Autodesk Inventor part; units mm, degrees
ref_plane "Start plane" through (0, 0, -25) normal (0, 0, 1) x (1, 0, 0)
ref_plane "End plane" through (0, 0, 2335) normal (0, 0, 1) x (1, 0, 0)
ref_plane "Work Plane4" through (0, 21, -25) normal (0, 0, -1) x (-1, 0, 0)
ref_plane "Start plane" through (0, 0, -25) normal (0, 0, 1) x (1, 0, 0)
ref_plane "End plane" through (0, 0, 2335) normal (0, 0, 1) x (1, 0, 0)
sketch "Sketch" plane through (0, 0, 0) normal (0, 0, 1) x (1, 0, 0)
  line L0 (-25, -21) -> (-25, 21)
  line L1 (-21, 25) -> (21, 25)
  line L2 (25, 21) -> (25, -21)
  line L3 (21, -25) -> (-21, -25)
  arc A0 (-25, -21) -> (-21, -25) centre (-21, -21) ccw
  arc A1 (25, 21) -> (21, 25) centre (21, 21) ccw
  arc A2 (-21, 25) -> (-25, 21) centre (-21, 21) ccw
  arc A3 (21, -25) -> (25, -21) centre (21, -21) ccw
  arc A4 (-21, 23) -> (-23, 21) centre (-21, 21) ccw
  line L4 (-21, 23) -> (21, 23)
  arc A5 (23, 21) -> (21, 23) centre (21, 21) ccw
  line L5 (23, 21) -> (23, -21)
  arc A6 (21, -23) -> (23, -21) centre (21, -21) ccw
  line L6 (21, -23) -> (-21, -23)
  arc A7 (-23, -21) -> (-21, -23) centre (-21, -21) ccw
  line L7 (-23, -21) -> (-23, 21)
  line L8 (0, 36.4497) -> (0, -36.4497) construction
  line L9 (-36.4497, 0) -> (36.4497, 0) construction
  dimension "d7" = 4
  dimension "d9" = 50
  dimension "d11" = 50
  dimension "d12" = 2
  dimension "d15" = 25
  dimension "d16" = 25
extrude "Body" add sketch "Sketch" along normal up to surface (2360 mm away) from surface at -25
sketch "Sketch3" plane through (0, 0, 0) normal (0, 0, 1) x (1, 0, 0)
  line L0 (0, 0) -> (10, 0)
ref_plane "Work Plane3" through (0, 0, 0) normal (0, -1, 0) x (1, 0, 0)
sketch "Sketch4" plane through (0, 0, 0) normal (0, -1, 0) x (1, 0, 0)
  line L0 (-2, -25) -> (12, -25)
  line L1 (-2, 2335) -> (12, 2335)
  dimension "d18" = 2360
ref_plane "Work Plane4" through (0, 21, -25) normal (0, 0, -1) x (-1, 0, 0)
split "Split1" plane through (0, 21, -25) removes the side toward (0, 0, -1)
ref_plane "Work Plane5" through (0, -21, 2335) normal (0, 0, 1) x (1, 0, 0)
split "Split2" plane through (0, -21, 2335) removes the side toward (0, 0, 1)
sketch "Sketch6" plane through (-25, 21, -25) normal (-1, 0, 0) x (0, 0, 1)
  line L0 (2360, 0) -> (0, 0)
  line L1 (0, 0) -> (2360, 0)
  line L2 (1180, 0) -> (1180, -42)
  line L3 (1160, -6) -> (1200, -6)
  line L4 (1200, -6) -> (1200, -36)
  line L5 (1200, -36) -> (1160, -36)
  line L6 (1160, -36) -> (1160, -6)
  line L7 (2360, -42) -> (0, -42)
  line L8 (1180, -21) -> (1190.0691, -21)
  point P0 (25, -21)
  dimension "d19" = 40
  dimension "d20" = 30
hole "Hole1" at (-25, 15, 1135) at (-25, -15, 1135) at (-25, -15, 1175) at (-25, 15, 1175) direction (1, 0, 0) diameter 5.5 end through all
equation "\"d7\" = G_IR"
equation "\"d9\" = G_W"
equation "\"d11\" = G_H"
equation "\"d12\" = G_T"
equation "\"d15\" = 0.5 * d9"
equation "\"d16\" = 0.5 * d11"
equation "\"d3\" = G_L"
equation "\"G_W\" = 50"
equation "\"G_H\" = 50"
equation "\"G_T\" = 2"
equation "\"G_IR\" = 4"
equation "\"G_L\" = d18"
equation "\"G_OFFSET_START\" = 25"
equation "\"G_OFFSET_END\" = 25"
equation "\"d13\" = -G_OFFSET_START"
equation "\"d14\" = G_OFFSET_END + B_L"
properties part number "ISO 10799-2 - 50x50x2 - 2360" material "Steel, Galvanized"
Geometry: final body of the model. Coordinates: model frame, mm. A direction names the side the tool comes from. Coordinates: 2 decimals unless noted, no trailing zeros. Order: outer loops, then holes, each group sorted by start corner. A loop starts at its lowest first (then second) coordinate and runs counter-clockwise, first axis right, second up. Notation, with made-up numbers: (43.25, 2.25) -> (62.25, 2.25) arc R19 ccw to (62.25, 14.25) -> close; hole circle Ø3 at (87, -18). An arc over 180 degrees is marked (long way). Write item = value, one per line.
(1) Line query: line 1 (Z direction, x = -24.2, y = 15); line 2 (Y direction, x = 24.2, z = 1175); line 3 (Y direction, x = 24.3, z = 1135). Output: solid intervals per line, ascending.
Solved:
line_1 = -25 to 1132.25, 1137.75 to 1172.25, 1177.75 to 2335
line_2 = -23.4 to -17.75, -12.25 to 12.25, 17.75 to 23.4
line_3 = -23.26 to -17.75, -12.25 to 12.25, 17.75 to 23.26
(2) Cut plane A-A on y = 2. Return loops of the section in (x, z), plus the area to 3 significant figures.
Solved:
outline = (-25, -25) -> (-23, -25) -> (-23, 2335) -> (-25, 2335) -> close; (23, -25) -> (25, -25) -> (25, 2335) -> (23, 2335) -> close
area = 9,440 mm²
(3) Access query for faces 5 (the flat face through (0, -25, 1138)), 6 (the flat face through (-23, 0, 1138)). Directions: +Z, -Z, +X, -X, +Y, -Y. A direction counts if a zero-diameter tool reaches every point of the face in a straight line with its end or side. Return the directions, or none.
Solved:
face_5 = +Z, -Z, +X, -X, -Y
face_6 = +Z, -Z
(4) Cut plane B-B on z = 600.5. Return loops of the section in (x, y).
Solved:
outline = (-25, -21) arc R4 ccw to (-21, -25) -> (21, -25) arc R4 ccw to (25, -21) -> (25, 21) arc R4 ccw to (21, 25) -> (-21, 25) arc R4 ccw to (-25, 21) -> close; hole (-23, -21) arc R2 ccw to (-21, -23) -> (21, -23) arc R2 ccw to (23, -21) -> (23, 21) arc R2 ccw to (21, 23) -> (-21, 23) arc R2 ccw to (-23, 21) -> close
(5) Pull-direction query (X, two-part tool) for faces 1 (the flat face through (0, 23, 1138)), 2 (the flat face through (0, 25, 1138)), 3 (the flat face through (25, 0, 1138)), 4 (the flat face through (-25, 0, 1138)); classes: pulls with the +X half, pulls with the -X half, needs draft (parallel to the pull), parting line crosses it, or undercut.
Solved:
face_1 = undercut
face_2 = needs draft
face_3 = pulls with the +X half
face_4 = pulls with the -X half
